Build history of the part. All positions in model axes, mm. Face numbers are marked on the shaded views. A direction names the side the tool comes from. Give positions to 0.01 mm unless a question says otherwise; leave off trailing zeros. Order: outer loops, then holes, each group sorted by start corner. A loop starts at its lowest first (then second) coordinate and runs counter-clockwise, first axis right, second up. Notation, with made-up numbers: (30, 45) - (75, 45) arc R19 ccw to (75, 52) - close; hole circle Ø7 at (-22, 1). An arc over 180 degrees is marked (long way). Answer in a Markdown table with one row per item.
```python
from build123d import *

# Parameters (mm, degrees)
RESSALTO_EXTRUS_O1_DEPTH = 15
ESBO_O2_R                = 1.8
CORTE_EXTRUS_O1_DEPTH    = 33.592176975
FILETE1_R                = 0.2
ESBO_O3_W                = 6
ESBO_O3_H                = 3
RESSALTO_EXTRUS_O2_DEPTH = 3
CORTE_EXTRUS_O2_DEPTH    = 2.8


with BuildPart() as part:
    # Esboço1 → Ressalto-extrusão1 (new, symmetric)
    with BuildSketch(Plane.XY):
        with BuildLine():
            Line((-22.5, 0), (22.5, 0))
            Line((22.5, 0), (28.5, 0))
            Line((28.5, 0), (28.5, 5))
            Line((28.5, 5), (22.5, 5))
            ThreePointArc((22.5, 5), (18.75, 1.25), (15, 5))
            ThreePointArc((15, 5), (11.25, 1.25), (7.5, 5))
            ThreePointArc((7.5, 5), (3.75, 1.25), (0, 5))
            ThreePointArc((0, 5), (-3.75, 1.25), (-7.5, 5))
            ThreePointArc((-7.5, 5), (-11.25, 1.25), (-15, 5))
            ThreePointArc((-15, 5), (-18.75, 1.25), (-22.5, 5))
            Line((-22.5, 5), (-28.5, 5))
            Line((-28.5, 5), (-28.5, 0))
            Line((-28.5, 0), (-22.5, 0))
        make_face()
    extrude(amount=RESSALTO_EXTRUS_O1_DEPTH, both=True)

    # Esboço2 → Corte-extrusão1 (cut, through all)
    with BuildSketch(Plane(origin=(0, 5, 0), x_dir=(1, 0, 0), z_dir=(0, 1, 0))):
        with Locations(Location((-25.5, 0, 0), (0, 0, 180))):
            Circle(ESBO_O2_R)
        with Locations((25.5, 0)):
            Circle(ESBO_O2_R)
    extrude(amount=-CORTE_EXTRUS_O1_DEPTH, mode=Mode.SUBTRACT)

    # Filete1
    filete1_edges = [part.edges().sort_by_distance(p)[0] for p in [
        (-15, 5, 0),
        (-7.5, 5, 0),
        (0, 5, 0),
        (7.5, 5, 0),
        (15, 5, 0),
    ]]
    fillet(filete1_edges, radius=FILETE1_R)

    # Esboço3 → Ressalto-extrusão2 (add)
    with BuildSketch(Plane(origin=(0, 5, 0), x_dir=(1, 0, 0), z_dir=(0, 1, 0))):
        with Locations((-25.5, 13.5)):
            Rectangle(ESBO_O3_W, ESBO_O3_H)
        with Locations((-25.5, -13.5)):
            Rectangle(ESBO_O3_W, ESBO_O3_H)
        with Locations((25.5, -13.5)):
            Rectangle(ESBO_O3_W, ESBO_O3_H)
        with Locations((25.5, 13.5)):
            Rectangle(ESBO_O3_W, ESBO_O3_H)
    extrude(amount=RESSALTO_EXTRUS_O2_DEPTH)

    # Esboço4 → Corte-extrusão2 (cut)
    with BuildSketch(Plane.XZ):
        Polygon((-29.021836642, 0), (-27.260918321, -3.05), (-23.739081679, -3.05), (-21.978163358, 0), (-23.739081679, 3.05), (-27.260918321, 3.05), align=None)
        Polygon((27.260918321, 3.05), (29.021836642, 0), (27.260918321, -3.05), (23.739081679, -3.05), (21.978163358, 0), (23.739081679, 3.05), align=None)
    extrude(amount=-CORTE_EXTRUS_O2_DEPTH, mode=Mode.SUBTRACT)


solid = part.part
```
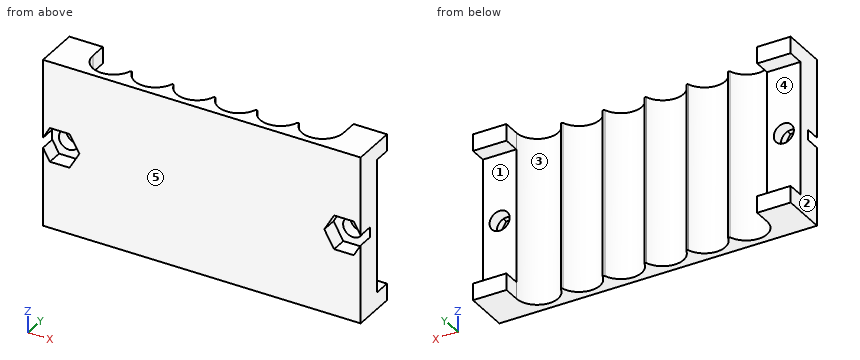
1. Cut at C-C on x = 11. Write the cut outline in (y, z), and give its area (3 significant figures).
Check result:
| item | result |
|---|---|
| outline | (0, -15) - (1.26, -15) - (1.26, 15) - (0, 15) - close |
| area | 37.8 mm² |
2. Two-plate mould, pull along X, no slides. Class the marked faces 1, 2 and 3: +X half, -X half, draft (parallel to the pull), parting line (faces both ways), or undercut.
Check result:
| item | result |
|---|---|
| face 1 | draft |
| face 2 | -X half |
| face 3 | undercut |
3. Probe line 1 (Z direction, x = 25.5, y = 4.45); line 2 (Z direction, x = -23, y = 7.75); line 3 (X direction, y = 5, z = -12.5). List the from-to ranges inside material, lowest first.
Check result:
| item | result |
|---|---|
| line 1 | z = -15 to -1.8, 1.8 to 15 |
| line 2 | z = -15 to -12, 12 to 15 |
| line 3 | x = -28.5 to -22.5, 22.5 to 28.5 |
4. Which spindle directions (+Z, -Z, +X, -X, +Y, -Y) get a long thin tool onto all of the face, cutting with end or side? Do the marked faces 4 and 5. Say none if no direction does.
Check result:
| item | result |
|---|---|
| face 4 | +X, -X, +Y |
| face 5 | +Z, -Z, +X, -X, -Y |
5. Cut at A-A on x = -25.5. Write the cut outline in (y, z).
Check result:
| item | result |
|---|---|
| outline | (0, -15) - (8, -15) - (8, -12) - (5, -12) - (5, -1.8) - (2.8, -1.8) - (2.8, -3.05) - (0, -3.05) - close; (0, 3.05) - (2.8, 3.05) - (2.8, 1.8) - (5, 1.8) - (5, 12) - (8, 12) - (8, 15) - (0, 15) - close |
6. Cut at B-B on y = 6. Write the cut outline in (x, z).
Check result:
| item | result |
|---|---|
| outline | (-28.5, -15) - (-22.5, -15) - (-22.5, -12) - (-28.5, -12) - close; (-28.5, 12) - (-22.5, 12) - (-22.5, 15) - (-28.5, 15) - close; (22.5, -15) - (28.5, -15) - (28.5, -12) - (22.5, -12) - close; (22.5, 12) - (28.5, 12) - (28.5, 15) - (22.5, 15) - close |
7. Drop flat-ended pins along their axis: P1, Ø1.8, axis at x = 24, z = -1.5, coming from the -Y side; P2, Ø5, axis at x = -25, z = 3, coming from the +Y side. Give the stop position or say it passes through.
Check result:
| item | result |
|---|---|
| P1 | stops at y = 2.8 |
| P2 | stops at y = 5 |
